CAD build for the part. Positions are in the model's coordinates, mm. Give positions to 0.01 mm unless a question says otherwise; leave off trailing zeros. Order: outer loops, then holes, each group sorted by start corner. A loop starts at its lowest first (then second) coordinate and runs counter-clockwise, first axis right, second up.
Item 1: Flat gauge pin, fed straight in: P1, Ø1.5, axis at x = -15.5, z = 1, coming from the +Y side. Where does the tip first touch, or does it go through?
Item 2: Band-saw the part on C-C on z = 1.25. Give the cut face in (x, y).
Item 3: Band-saw the part on B-B on y = 61. Give the cut face in (x, z) (3 decimals).
Item 4: Wall check: L1, parallel to X at y = 54.5, z = 3; L2, parallel to Y at x = 0, z = 0.3; L3, parallel to Y at x = 9.5, z = 1.05. Give the ranges that are in metal, low to high.
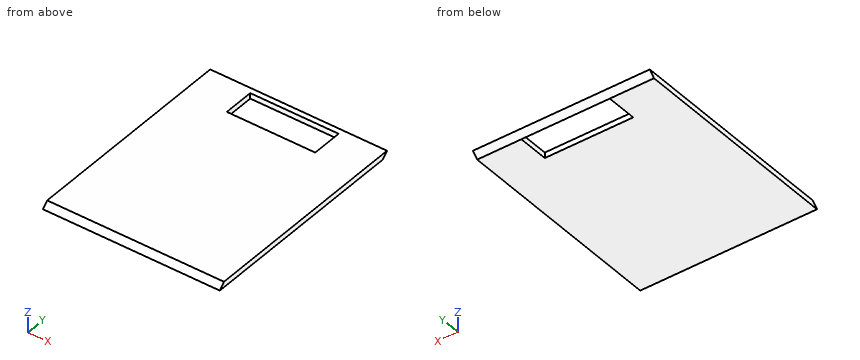
```python
from build123d import *

# Parameters (mm, degrees)
F0_W     = 101.6
F0_H     = 127
F1_DEPTH = 3.175
F2_SIZE  = 3.17499
F3_SIZE  = 3.17499
F4_W     = 31.75
F4_H     = 17.7633663237
F4_W_2   = 19.05
F5_DEPTH = 3.175


# Not quite as in the source:
# - a fillet or chamfer is up to 0.001 mm smaller than in the source, because OpenCascade refuses the exact size
# - a length typed as a fraction of an inch, garbled in the dataset ("3 / 203.2 mm" for 3/8 in), is restored


with BuildPart() as f1:
    # F0 (on Top) → F1 (new body)
    with BuildSketch(Plane.XY):
        with Locations((5.2556597352, 10.8384059966)):
            Rectangle(F0_W, F0_H)
    extrude(amount=F1_DEPTH)

    # F2 (size 3.175 in the source; OpenCascade refuses exactly that, so slightly less here)
    f2_edges = [f1.edges().sort_by_distance(p)[0] for p in [
        (5.25566, 74.338406, 0),
    ]]
    chamfer(f2_edges, length=F2_SIZE)

    # F3 (size 3.175 in the source; OpenCascade refuses exactly that, so slightly less here)
    f3_edges = [f1.edges().sort_by_distance(p)[0] for p in [
        (5.25566, -52.661594, 3.175),
    ]]
    chamfer(f3_edges, length=F3_SIZE)

    # F4 (on face) → F5 (cut)
    with BuildSketch(Plane(origin=(0, 0, 0), x_dir=(1, 0, 0), z_dir=(0, 0, -1))):
        with Locations((-4.2693402648, -62.2817228347)):
            Rectangle(F4_W, F4_H)
        with Locations((21.1306597352, -62.2817228347)):
            Rectangle(F4_W_2, F4_H)
    extrude(amount=-F5_DEPTH, mode=Mode.SUBTRACT)


solid = f1.part
```
The answers:
1. P1: stops at y = 72.91
2. outline: (-45.54, -51.41) - (56.06, -51.41) - (56.06, 72.41) - (-45.54, 72.41) - close; hole (-20.14, 53.4) - (30.66, 53.4) - (30.66, 71.16) - (-20.14, 71.16) - close
3. outline: (-45.544, 0) - (-20.144, 0) - (-20.144, 3.175) - (-45.544, 3.175) - close; (30.656, 0) - (56.056, 0) - (56.056, 3.175) - (30.656, 3.175) - close
4. L1: x = -45.54 to -20.14, 30.66 to 56.06
4. L2: y = -52.36 to 53.4, 71.16 to 71.46
4. L3: y = -51.61 to 53.4, 71.16 to 72.21
